Autodesk Fusion 360 part; units mm, degrees
sketch "Sketch1" plane through (0, 0, 0) normal (0, 0, 1) x (1, 0, 0)
  line L0 (0, 0) -> (55, 0)
  line L1 (55, 0) -> (55, 55)
  line L2 (55, 55) -> (0, 55)
  line L3 (0, 55) -> (0, 0)
  line L4 (55, 55) -> (45, 55)
  line L5 (45, 55) -> (45, 47)
  line L6 (45, 47) -> (55, 47)
  line L7 (55, 47) -> (55, 55)
  line L8 (0, 0) -> (10, 0)
  line L9 (10, 0) -> (10, 8)
  line L10 (10, 8) -> (0, 8)
  line L11 (0, 8) -> (0, 0)
  line L12 (0, 8) -> (55, 8)
  line L13 (55, 8) -> (55, 47)
  line L14 (55, 47) -> (0, 47)
  line L15 (0, 47) -> (0, 8)
  circle A0 centre (5, 5) radius 1.75
  circle A1 centre (50, 50) radius 1.75
  line L16 (0, 10) -> (55, 10)
  line L17 (55, 10) -> (55, 45)
  line L18 (55, 45) -> (0, 45)
  line L19 (0, 45) -> (0, 10)
  dimension "d1" = 55
  dimension "d7" = 3.5
  dimension "d8" = 3.5
  dimension "d9" = 5
  dimension "d11" = 5
  dimension "d47" = 39
  dimension "d48" = 55
  dimension "d49" = 35
  dimension "d50" = 2
  dimension "d53" = 5
  dimension "d54" = 5
  dimension "d55" = 8
  dimension "d56" = 8
  dimension "d57" = 10
  dimension "d58" = 10
extrude "Extrude1" add sketch "Sketch1" along normal blind 2 contours L0 L3 L8 L9 L10 L11 L12 | L1 L3 L10 L12 L13 L15 L16 | L1 L3 L13 L15 L16 L17 L18 L19 | L1 L3 L6 L13 L14 L15 L18 | L1 L2 L4 L5 L6 L7 L14
sketch "Sketch2" plane through (0, 0, 2) normal (0, 0, 1) x (-1, 0, 0)
  circle A0 centre (-50, -50) radius 1.75
  circle A1 centre (-5, -5) radius 1.75
  line L0 (0, -47) -> (0, 0)
  line L1 (0, 0) -> (-10, 0)
  line L2 (-10, 0) -> (-10, -8)
  line L3 (-10, -8) -> (-55, -8)
  line L4 (-55, -8) -> (-55, -55)
  line L5 (-55, -55) -> (-45, -55)
  line L6 (-45, -55) -> (-45, -47)
  line L7 (-45, -47) -> (0, -47)
  circle A2 centre (-5, -5) radius 1.875
  circle A3 centre (-50, -50) radius 1.875
  line L8 (-4.0912, -23.3213) -> (-51.331, -24.5146) construction
  line L9 (-51.331, -24.5146) -> (-51.1199, -32.872) construction
  line L10 (-51.1199, -32.872) -> (-3.8801, -31.6787) construction
  line L11 (-3.8801, -31.6787) -> (-4.0912, -23.3213) construction
  line L12 (0, -47) -> (0, -8)
  line L13 (0, -8) -> (-55, -8)
  dimension "d15" = 3.75
  dimension "d40" = 5
  dimension "d41" = 27.5
  dimension "d42" = 19.5
hole "Hole1" at (50, 50, 2) direction (0, 0, -1) diameter 3.5 depth 2 tip angle 118
hole "Hole2" at (5, 5, 2) direction (0, 0, -1) diameter 3.5 depth 2 tip angle 118
fillet "Fillet1" radius 1 1 edges at (0, 47, 1)
fillet "Fillet2" radius 1 1 edges at (45, 55, 1)
fillet "Fillet3" radius 1 1 edges at (45, 47, 1)
fillet "Fillet4" radius 1 1 edges at (55, 55, 1)
fillet "Fillet5" radius 1 2 edges at (0, 0, 1) (10, 0, 1)
fillet "Fillet6" radius 1 1 edges at (10, 8, 1)
fillet "Fillet7" radius 1 1 edges at (55, 8, 1)
emboss "Emboss1" [suppressed]
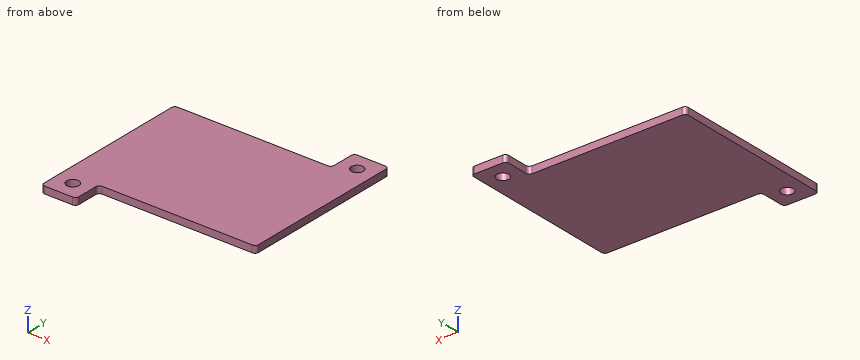
The listing builds one solid part. Answer for the finished solid, in the listing's coordinates (mm). Coordinates: 2 decimals unless noted, no trailing zeros. Write each loop counter-clockwise with the first axis right and the second up, starting at its lowest first coordinate (ties: lowest second). Pieces come first, ordered by that corner, then holes. Notation, with made-up numbers: M 17.25,-10.5 L 23.25,-10.5 A11 cw 23.25,9.5 Z; hole C 32,-37.5 d7. An arc over 180 degrees is marked long. Put each result on its own line as item: value. Start each with the question number.
1. A cutting plane is placed at C-C on y = 50. Write down the section's boundary in (x, z).
2. A cutting plane is placed at A-A on z = 0.85. Write down the section's boundary in (x, y).
3. Consider line 1 (X direction, y = 5, z = 0.4); line 2 (X direction, y = 50, z = 0.75); line 3 (Y direction, x = 50, z = 0.5). Determine where each line is inside the solid, lowest interval first. Write a range as from..to.
4. A cutting plane is placed at B-B on x = 5. Write down the section's boundary in (y, z), then the cut area to 3 significant figures.
5. A cutting plane is placed at D-D on x = 16.5. Write down the section's boundary in (y, z).
6. Flat-ended cylindrical pins translate along their axes: P1, Ø2, axis at x = 17, y = 38.5, coming from the -Z side; P2, Ø3, axis at x = 50, y = 50, coming from the -Z side; P3, Ø1, axis at y = 3, z = 1, coming from the +X side; P4, Ø1, axis at x = 25, z = 1, coming from the +Y side. Find the tip coordinate at first contact, or state that the pin passes through.
Resolved:
1. outline: M 45,0 L 48.25,0 L 48.25,2 L 45,2 Z; M 51.75,0 L 55,0 L 55,2 L 51.75,2 Z
2. outline: M 0,1 A1 ccw 1,0 L 9,0 A1 ccw 10,1 L 10,7 A1 cw 11,8 L 54,8 A1 ccw 55,9 L 55,54 A1 ccw 54,55 L 46,55 A1 ccw 45,54 L 45,48 A1 cw 44,47 L 1,47 A1 ccw 0,46 Z; hole C 5,5 d3.5; hole C 50,50 d3.5
3. line 1: x = 0..3.25, 6.75..10
3. line 2: x = 45..48.25, 51.75..55
3. line 3: y = 8..48.25, 51.75..55
4. outline: M 0,0 L 3.25,0 L 3.25,2 L 0,2 Z; M 6.75,0 L 47,0 L 47,2 L 6.75,2 Z
4. area: 87.0 mm2
5. outline: M 8,0 L 47,0 L 47,2 L 8,2 Z
6. P1: stops at z = 0
6. P2: passes through
6. P3: stops at x = 10
6. P4: stops at y = 47
